Autodesk Inventor part; units mm, degrees
ref_plane "YZ Plane" through (0, 0, 0) normal (1, 0, 0) x (0, 1, 0)
ref_plane "XZ Plane" through (0, 0, 0) normal (0, 1, 0) x (-1, 0, 0)
ref_plane "XY Plane" through (0, 0, 0) normal (0, 0, 1) x (1, 0, 0)
sketch "Sketch2" plane through (0, 0, 0) normal (0, 0, 1) x (1, 0, 0)
  line L0 (-75, -25) -> (75, -25)
  line L1 (75, -25) -> (75, 25)
  line L2 (75, 25) -> (-75, 25)
  line L3 (-75, 25) -> (-75, -25)
  line L4 (-75, -25) -> (75, 25) construction
  line L5 (75, -25) -> (-75, 25) construction
  point P0 (0, 0)
  dimension "d1" = 150
  dimension "d2" = 50
extrude "Extrusion1" add sketch "Sketch2" along normal mid plane 10
sketch "Sketch3" plane through (0, 0, 5) normal (0, 0, 1) x (1, 0, 0)
  line L0 (-75, 25) -> (-75, -25)
  line L1 (75, 25) -> (-75, 25)
  point P0 (0, 0)
  point P1 (-65, 0)
  dimension "d40" = 10
  dimension "d43" = 25
hole "Hole1" at (-65, 0, 5) direction (0, 0, -1) diameter 4.134 depth 14.2 tip angle 118
sketch "Sketch4" plane through (0, 0, 5) normal (0, 0, 1) x (1, 0, 0)
  line L0 (-75, 25) -> (-75, -25)
  line L1 (75, 25) -> (-75, 25)
  point P0 (0, 0)
  point P1 (-45, 5)
  dimension "d41" = 30
  dimension "d42" = 20
hole "Hole2" at (-45, 5, 5) direction (0, 0, -1) diameter 4.917 depth 17.1 tip angle 118
sketch "Sketch5" plane through (0, 0, 5) normal (0, 0, 1) x (1, 0, 0)
  line L0 (-75, 25) -> (-75, -25)
  line L1 (75, 25) -> (-75, 25)
  point P0 (0, 0)
  point P1 (-25, 5)
  dimension "d44" = 50
  dimension "d45" = 20
hole "Hole3" at (-25, 5, 5) direction (0, 0, -1) diameter 6.647 depth 22.2 tip angle 118
sketch "Sketch6" plane through (0, 0, 5) normal (0, 0, 1) x (1, 0, 0)
  line L0 (-75, 25) -> (-75, -25)
  line L1 (75, 25) -> (-75, 25)
  point P0 (0, 0)
  point P1 (5, 5)
  dimension "d46" = 80
  dimension "d47" = 20
hole "Hole4" at (5, 5, 5) direction (0, 0, -1) diameter 6 depth 14.2 tip angle 118
sketch "Sketch7" plane through (0, 0, 5) normal (0, 0, 1) x (1, 0, 0)
  line L0 (-75, 25) -> (-75, -25)
  line L1 (75, 25) -> (-75, 25)
  point P0 (0, 0)
  point P1 (25, 5)
  dimension "d48" = 100
  dimension "d49" = 20
hole "Hole5" at (25, 5, 5) direction (0, 0, -1) diameter 10 depth 14.2 tip angle 118
sketch "Sketch8" plane through (0, 0, 5) normal (0, 0, 1) x (1, 0, 0)
  point P0 (0, 0)
  point P1 (51.0965, 5.234)
hole "Hole6" at (51.0965, 5.234, 5) direction (0, 0, -1) diameter 17.294 depth 51.2 tip angle 118
properties part number "홀간 거리 확인 파트-2" material "SS400"
Here's how the part is built. I have some questions about the finished solid (model axes, mm). Give positions to 0.01 mm unless a question says otherwise; leave off trailing zeros. Loops run counter-clockwise (first coordinate to the right, second up) from the corner with the lowest first, then second, coordinate; pieces in that order, holes last. Notation, with made-up numbers: (23, 6) -> (48, 6) arc R33 ccw to (48, 37) -> close; hole circle Ø8 at (83, 62). An arc over 180 degrees is marked (long way). Use one line per item in the form item = value. Start each with the question number.
1) Imagine slicing it at C-C (z = -2.5). Please give me the cut outline in (x, y), then the cut area to 3 significant figures.
2) Imagine slicing it at B-B (y = 5). Please give me the cut outline in (x, z).
3) For P1, Ø5, axis at x = 5, y = 5, coming from the -Z side, with a flat end and sliding along its axis, tell me the tip position at first contact or that it passes through.
4) Thinking about a two-plate mould opening in X: for faces 1 (the face through (-28.3, 5.4, -0.1)), 2 (the face through (75, 0, 0)), 3 (the face through (-75, 0, 0)), 4 (the face through (-1, 0, 5)), which applies, +X half, -X half, draft (parallel to the pull), parting line (faces both ways), or undercut?
5) Please list where these lines run through material, in increasing order: line 1 along X through (y, z) = (5, 1); line 2 along Y through (x, z) = (5, 1.25); line 3 along X through (y, z) = (1, 2).
6) Imagine slicing it at A-A (x = 5). Please give me the cut outline in (y, z), then the cut area to 3 significant figures.
7) Imagine slicing it at D-D (x = -45). Please give me the cut outline in (y, z).
Check values:
q1.outline = (-75, -25) -> (75, -25) -> (75, 25) -> (-75, 25) -> close; hole circle Ø4.13 at (-65, 0); hole circle Ø4.92 at (-45, 5); hole circle Ø6.65 at (-25, 5); hole circle Ø6 at (5, 5); hole circle Ø10 at (25, 5); hole circle Ø17.29 at (51.1, 5.23)
q1.area = 7,090 mm^2
q2.outline = (-75, -5) -> (-47.46, -5) -> (-47.46, 5) -> (-75, 5) -> close; (-42.54, -5) -> (-28.32, -5) -> (-28.32, 5) -> (-42.54, 5) -> close; (-21.68, -5) -> (2, -5) -> (2, 5) -> (-21.68, 5) -> close; (8, -5) -> (20, -5) -> (20, 5) -> (8, 5) -> close; (30, -5) -> (42.45, -5) -> (42.45, 5) -> (30, 5) -> close; (59.74, -5) -> (75, -5) -> (75, 5) -> (59.74, 5) -> close
q3.P1 = through
q4.face_1 = undercut
q4.face_2 = +X half
q4.face_3 = -X half
q4.face_4 = draft
q5.line_1 = -75 to -47.46, -42.54 to -28.32, -21.68 to 2, 8 to 20, 30 to 42.45, 59.74 to 75
q5.line_2 = -25 to 2, 8 to 25
q5.line_3 = -75 to -66.81, -63.19 to 22, 28 to 43.56, 58.64 to 75
q6.outline = (-25, -5) -> (2, -5) -> (2, 5) -> (-25, 5) -> close; (8, -5) -> (25, -5) -> (25, 5) -> (8, 5) -> close
q6.area = 440 mm^2
q7.outline = (-25, -5) -> (2.54, -5) -> (2.54, 5) -> (-25, 5) -> close; (7.46, -5) -> (25, -5) -> (25, 5) -> (7.46, 5) -> close
